Verification items for the finished model (mm, model axes). A direction names the side the tool comes from. Give positions to 0.01 mm unless a question says otherwise; leave off trailing zeros. Order: outer loops, then holes, each group sorted by start corner. A loop starts at its lowest first (then second) coordinate and runs counter-clockwise, first axis right, second up. Notation, with made-up numbers: (83, 63) -> (110, 63) arc R25 cw to (110, 84) -> close; hole circle Ø6 at (57.5, -1.75). An arc over 180 degrees is marked (long way). Return JSON: item names as keys, results as strings. Group by question number.
(1) Tool access check on faces 4 (the face through (210.4, -75.8, -1.7)), 5 (the face through (209.155, -51.479, 0.556)), 6 (the face through (126.836, -65, 0)). Record the directions out of +Z, -Z, +X, -X, +Y, -Y that give a thin tool (end or side, any length) a straight path to the whole face; none if there is none.
(2) Cross-section at C-C on y = -104. Enter the section's corners in (x, z).
(3) Cross-section at B-B on x = 166.5. Enter the section's corners in (y, z).
(4) Depth check by flat-ended pin: pin 1 Ø1 at (x, y) = (187.5, -77.5) entering from -Z; pin 2 Ø9 at (x, y) = (90, -63) entering from -Z; pin 3 Ø1.2 at (y, z) = (-61.5, -1) entering from +X. Enter the tip coordinate at first touch or a pass-through.
(5) Thickness scan on line 1 along Y through (x, z) = (107, 3.15); line 2 along Y through (x, z) = (187, 1.9); line 3 along Y through (x, z) = (208, 1.75). Record the ranges inside material, lowest first.
(6) Cross-section at A-A on y = -74. Enter the section's corners in (x, z).
(7) Release check for a two-part mould opening along X. For faces 1 (the face through (210.21, -112.97, -1.73)), 2 (the face through (107.46, -116.05, 3.59)), 3 (the face through (150, -94, -1.5)) record: pulls with the +X half, pulls with the -X half, needs draft (parallel to the pull), parting line crosses it, or undercut.
from build123d import *

# Parameters (mm, degrees)
ESQUISSE2_W                = 132
ESQUISSE2_H                = 74
BOSS_EXTRU_1_DEPTH         = 4.5
BOSS_EXTRU_PWRSTAGES_DEPTH = 1.5
ENL_V_MAT_SELFS_DEPTH      = 1.25
ESQUISSE6_W                = 127.502
ESQUISSE6_H                = 30.958
BOSS_EXTRU_ASICS_DEPTH     = 1.5
ESQUISSE7_R                = 3
BOSS_EXTRU_FIXS_DEPTH      = 3.5
TROU_TARAUD_M31_D          = 2.5
TROU_TARAUD_M31_DEPTH      = 8
ESQUISSE15_R               = 2.1
ENL_V_MAT_EXTRU_1_DEPTH    = 5.5
ENL_V_START                = 3.5
ESQUISSE16_R               = 3.5
ENL_V_MAT_EXTRU_3_DEPTH    = 6.2


with BuildPart() as part:
    # Esquisse2 → Boss.-Extru.1 (new body)
    with BuildSketch(Plane.XY):
        with Locations((147, -83)):
            Rectangle(ESQUISSE2_W, ESQUISSE2_H)
    extrude(amount=BOSS_EXTRU_1_DEPTH)

    # Esquisse4 → Boss.-Extru. PWRstages (add)
    with BuildSketch(Plane(origin=(0, 0, 0), x_dir=(-1, 0, 0), z_dir=(0, 0, -1))):
        with BuildLine():
            Line((-190.85, -58), (-185.85, -58))
            ThreePointArc((-185.85, -58), (-184.435786438, -58.585786438), (-183.85, -60))
            Line((-183.85, -60), (-183.85, -64))
            ThreePointArc((-183.85, -64), (-184.435786438, -65.414213562), (-185.85, -66))
            Line((-185.85, -66), (-190.85, -66))
            ThreePointArc((-190.85, -66), (-192.264213562, -65.414213562), (-192.85, -64))
            Line((-192.85, -64), (-192.85, -60))
            ThreePointArc((-192.85, -60), (-192.264213562, -58.585786438), (-190.85, -58))
        make_face()
        with BuildLine():
            Line((-125.911169345, -57.999392956), (-120.911169345, -57.999392956))
            ThreePointArc((-120.911169345, -57.999392956), (-119.496955783, -58.585179394), (-118.911169345, -59.999392956))
            Line((-118.911169345, -59.999392956), (-118.911169345, -63.999392956))
            ThreePointArc((-118.911169345, -63.999392956), (-119.496955783, -65.413606518), (-120.911169345, -65.999392956))
            Line((-120.911169345, -65.999392956), (-125.911169345, -65.999392956))
            ThreePointArc((-125.911169345, -65.999392956), (-127.325382908, -65.413606518), (-127.911169345, -63.999392956))
            Line((-127.911169345, -63.999392956), (-127.911169345, -59.999392956))
            ThreePointArc((-127.911169345, -59.999392956), (-127.325382908, -58.585179394), (-125.911169345, -57.999392956))
        make_face()
        with BuildLine():
            Line((-158.396550345, -57.998313843), (-153.396550345, -57.998313843))
            ThreePointArc((-153.396550345, -57.998313843), (-151.982336782, -58.584100281), (-151.396550345, -59.998313843))
            Line((-151.396550345, -59.998313843), (-151.396550345, -63.998313843))
            ThreePointArc((-151.396550345, -63.998313843), (-151.982336782, -65.412527406), (-153.396550345, -65.998313843))
            Line((-153.396550345, -65.998313843), (-158.396550345, -65.998313843))
            ThreePointArc((-158.396550345, -65.998313843), (-159.810763907, -65.412527406), (-160.396550345, -63.998313843))
            Line((-160.396550345, -63.998313843), (-160.396550345, -59.998313843))
            ThreePointArc((-160.396550345, -59.998313843), (-159.810763907, -58.584100281), (-158.396550345, -57.998313843))
        make_face()
        with BuildLine():
            Line((-93.473877357, -58.003087947), (-88.473877357, -58.003087947))
            ThreePointArc((-88.473877357, -58.003087947), (-87.059663795, -58.588874385), (-86.473877357, -60.003087947))
            Line((-86.473877357, -60.003087947), (-86.473877357, -64.003087947))
            ThreePointArc((-86.473877357, -64.003087947), (-87.059663795, -65.417301509), (-88.473877357, -66.003087947))
            Line((-88.473877357, -66.003087947), (-93.473877357, -66.003087947))
            ThreePointArc((-93.473877357, -66.003087947), (-94.888090919, -65.417301509), (-95.473877357, -64.003087947))
            Line((-95.473877357, -64.003087947), (-95.473877357, -60.003087947))
            ThreePointArc((-95.473877357, -60.003087947), (-94.888090919, -58.588874385), (-93.473877357, -58.003087947))
        make_face()
    extrude(amount=BOSS_EXTRU_PWRSTAGES_DEPTH)

    # Esquisse3 → Enlèv. mat.-SELFs (cut, symmetric)
    with BuildSketch(Plane(origin=(0, 0, 0), x_dir=(-1, 0, 0), z_dir=(0, 0, -1))):
        with BuildLine():
            Line((-203.755, -59.925), (-193.755, -59.925))
            ThreePointArc((-193.755, -59.925), (-192.340786438, -60.510786438), (-191.755, -61.925))
            Line((-191.755, -61.925), (-191.755, -68.925))
            ThreePointArc((-191.755, -68.925), (-192.340786438, -70.339213562), (-193.755, -70.925))
            Line((-193.755, -70.925), (-203.755, -70.925))
            ThreePointArc((-203.755, -70.925), (-205.169213562, -70.339213562), (-205.755, -68.925))
            Line((-205.755, -68.925), (-205.755, -61.925))
            ThreePointArc((-205.755, -61.925), (-205.169213562, -60.510786438), (-203.755, -59.925))
        make_face()
        with BuildLine():
            Line((-171.301526488, -59.932281425), (-161.301526488, -59.932281425))
            ThreePointArc((-161.301526488, -59.932281425), (-159.887312925, -60.518067862), (-159.301526488, -61.932281425))
            Line((-159.301526488, -61.932281425), (-159.301526488, -68.932281425))
            ThreePointArc((-159.301526488, -68.932281425), (-159.887312925, -70.346494987), (-161.301526488, -70.932281425))
            Line((-161.301526488, -70.932281425), (-171.301526488, -70.932281425))
            ThreePointArc((-171.301526488, -70.932281425), (-172.71574005, -70.346494987), (-173.301526488, -68.932281425))
            Line((-173.301526488, -68.932281425), (-173.301526488, -61.932281425))
            ThreePointArc((-173.301526488, -61.932281425), (-172.71574005, -60.518067862), (-171.301526488, -59.932281425))
        make_face()
        with BuildLine():
            Line((-138.836257744, -59.927884864), (-128.836257744, -59.927884864))
            ThreePointArc((-128.836257744, -59.927884864), (-127.422044181, -60.513671302), (-126.836257744, -61.927884864))
            Line((-126.836257744, -61.927884864), (-126.836257744, -68.927884864))
            ThreePointArc((-126.836257744, -68.927884864), (-127.422044181, -70.342098426), (-128.836257744, -70.927884864))
            Line((-128.836257744, -70.927884864), (-138.836257744, -70.927884864))
            ThreePointArc((-138.836257744, -70.927884864), (-140.250471306, -70.342098426), (-140.836257744, -68.927884864))
            Line((-140.836257744, -68.927884864), (-140.836257744, -61.927884864))
            ThreePointArc((-140.836257744, -61.927884864), (-140.250471306, -60.513671302), (-138.836257744, -59.927884864))
        make_face()
        with BuildLine():
            Line((-106.349673037, -59.931395797), (-96.349673037, -59.931395797))
            ThreePointArc((-96.349673037, -59.931395797), (-94.935459474, -60.517182235), (-94.349673037, -61.931395797))
            Line((-94.349673037, -61.931395797), (-94.349673037, -68.931395797))
            ThreePointArc((-94.349673037, -68.931395797), (-94.935459474, -70.34560936), (-96.349673037, -70.931395797))
            Line((-96.349673037, -70.931395797), (-106.349673037, -70.931395797))
            ThreePointArc((-106.349673037, -70.931395797), (-107.763886599, -70.34560936), (-108.349673037, -68.931395797))
            Line((-108.349673037, -68.931395797), (-108.349673037, -61.931395797))
            ThreePointArc((-108.349673037, -61.931395797), (-107.763886599, -60.517182235), (-106.349673037, -59.931395797))
        make_face()
    extrude(amount=ENL_V_MAT_SELFS_DEPTH, both=True, mode=Mode.SUBTRACT)

    # Esquisse6 → Boss.-Extru. ASICs (add)
    with BuildSketch(Plane(origin=(0, 0, 0), x_dir=(-1, 0, 0), z_dir=(0, 0, -1))):
        with Locations((-149.249, -94.521)):
            Rectangle(ESQUISSE6_W, ESQUISSE6_H)
    extrude(amount=BOSS_EXTRU_ASICS_DEPTH)

    # Esquisse7 → Boss.-Extru. FIXs (add)
    with BuildSketch(Plane(origin=(0, 0, 0), x_dir=(-1, 0, 0), z_dir=(0, 0, -1))):
        with Locations((-208, -51)):
            Circle(ESQUISSE7_R)
        with Locations((-86, -51)):
            Circle(ESQUISSE7_R)
        with Locations((-86, -74)):
            Circle(ESQUISSE7_R)
        with Locations((-86, -115)):
            Circle(ESQUISSE7_R)
        with Locations((-208, -115)):
            Circle(ESQUISSE7_R)
        with Locations((-208, -74)):
            Circle(ESQUISSE7_R)
    extrude(amount=BOSS_EXTRU_FIXS_DEPTH)

    # Trou taraudé M31
    with Locations(Plane(origin=(0, 0, -3.5), x_dir=(-1, 0, 0), z_dir=(0, 0, -1))):
        with Locations((-208, -115), (-208, -74), (-208, -51), (-86, -51), (-86, -74), (-86, -115)):
            Hole(TROU_TARAUD_M31_D / 2, depth=TROU_TARAUD_M31_DEPTH)

    # Esquisse15 → Enlèv. mat.-Extru.1 (cut, through all)
    with BuildSketch(Plane(origin=(0, 0, 0), x_dir=(-1, 0, 0), z_dir=(0, 0, -1))):
        with Locations((-187, -52)):
            Circle(ESQUISSE15_R)
        with Locations((-107, -52)):
            Circle(ESQUISSE15_R)
        with Locations((-187, -114)):
            Circle(ESQUISSE15_R)
        with Locations((-107, -114)):
            Circle(ESQUISSE15_R)
    extrude(amount=-ENL_V_MAT_EXTRU_1_DEPTH, mode=Mode.SUBTRACT)

    # Esquisse16 → Enlèv. mat.-Extru.3 (cut)
    with BuildSketch(Plane(origin=(0, 0, 0), x_dir=(-1, 0, 0), z_dir=(0, 0, -1)).offset(ENL_V_START)):
        with Locations((-187, -52)):
            Circle(ESQUISSE16_R)
        with Locations((-107, -52)):
            Circle(ESQUISSE16_R)
        with Locations((-107, -114)):
            Circle(ESQUISSE16_R)
        with Locations((-187, -114)):
            Circle(ESQUISSE16_R)
    extrude(amount=-ENL_V_MAT_EXTRU_3_DEPTH, mode=Mode.SUBTRACT)


solid = part.part
Verdict:
{
 "1": {"face 4": "-Z", "face 5": "+Z, -Z", "face 6": "none"},
 "2": {"outline": "(81, 0) -> (85.5, 0) -> (85.5, -1.5) -> (213, -1.5) -> (213, 4.5) -> (81, 4.5) -> close"},
 "3": {"outline": "(-120, 0) -> (-110, 0) -> (-110, -1.5) -> (-79.04, -1.5) -> (-79.04, 0) -> (-70.93, 0) -> (-70.93, 1.25) -> (-59.93, 1.25) -> (-59.93, 0) -> (-46, 0) -> (-46, 4.5) -> (-120, 4.5) -> close"},
 "4": {"pin 1": "z = 0", "pin 2": "z = -1.5", "pin 3": "x = 192.85"},
 "5": {"line 1": "-120 to -116.1, -111.9 to -54.1, -49.9 to -46", "line 2": "-120 to -117.5, -110.5 to -55.5, -48.5 to -46", "line 3": "-120 to -116.25, -113.75 to -75.25, -72.75 to -52.25, -49.75 to -46"},
 "6": {"outline": "(81, 0) -> (83, 0) -> (83, -3.5) -> (84.75, -3.5) -> (84.75, 4.5) -> (81, 4.5) -> close; (87.25, -3.5) -> (89, -3.5) -> (89, 0) -> (205, 0) -> (205, -3.5) -> (206.75, -3.5) -> (206.75, 4.5) -> (87.25, 4.5) -> close; (209.25, -3.5) -> (211, -3.5) -> (211, 0) -> (213, 0) -> (213, 4.5) -> (209.25, 4.5) -> close"},
 "7": {"face 1": "undercut", "face 2": "undercut", "face 3": "needs draft"}
}
